Source: three-view drawing plus pictorial views. Frame: mm from the lowest corner of the part. A direction names the side the tool comes from. Give positions to 0.01 mm unless a question says otherwise; leave off trailing zeros. Write each loop counter-clockwise with the first axis right and the second up, starting at its lowest first coordinate (ties: lowest second). Pieces come first, ordered by that corner, then holes. Notation, with made-up numbers: (-33.75, 87) - (-9.75, 87) arc R28 cw to (-9.75, 113) - close; hole circle Ø2 at (74.25, -31.75). An arc over 180 degrees is marked (long way). One line per question, with ' | ' between items. Start each with the question number.
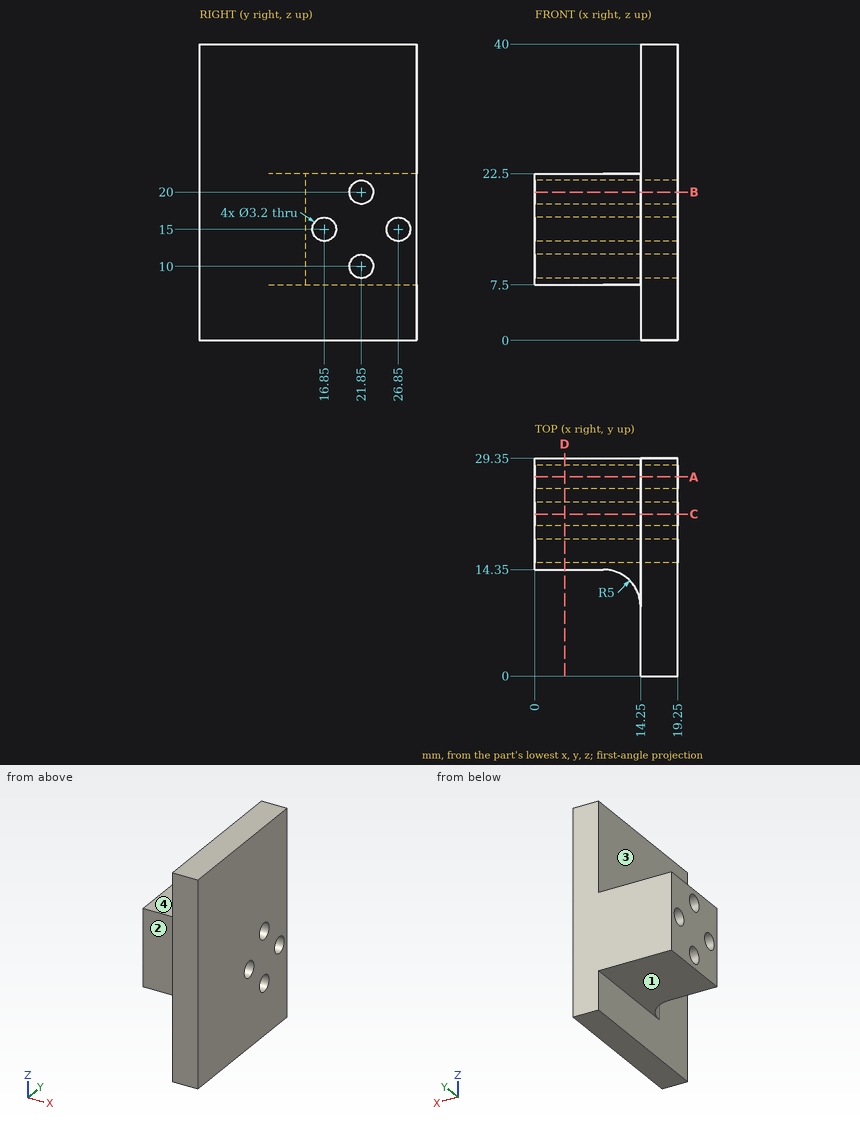
1) Reachability of the marked faces 1, 2, 3 and 4 from +Z, -Z, +X, -X, +Y, -Y: full face, straight path, thin tool, end or side. Return the list, or none.
2) Line query: L1, parallel to Y at x = 7, z = 15; L2, parallel to Y at x = 15.25, z = 15; L3, parallel to Z at x = 11, y = 22.5. Output: solid intervals per line, ascending.
3) Section D-D, the plane x = 4. Output: boundary loops of the cut face in (y, z), plus the area to 3 significant figures.
4) Section A-A, the plane y = 26.85. Output: boundary loops of the cut face in (x, z), plus the area to 3 significant figures.
5) First-contact query: pin 1 Ø3 at (y, z) = (23, 29) entering from -X; pin 2 Ø3 at (y, z) = (16.85, 15) entering from -X; pin 3 Ø7 at (x, y) = (5.5, 22) entering from -Z; pin 4 Ø8 at (x, y) = (3, 22.5) entering from +Z. Flat tips, straight axial feed; report the tip coordinate or a pass-through.
6) Section B-B, the plane z = 20. Output: boundary loops of the cut face in (x, y).
7) Section C-C, the plane y = 21.85. Output: boundary loops of the cut face in (x, z).
Answer key:
1) face 1: -Z, -X, +Y, -Y | face 2: +Z, -Z, -X, -Y | face 3: -X, -Y | face 4: +Z, -X, +Y, -Y
2) L1: 14.35 to 15.25, 18.45 to 25.25, 28.45 to 29.35 | L2: 0 to 15.25, 18.45 to 25.25, 28.45 to 29.35 | L3: 7.5 to 8.54, 11.46 to 18.54, 21.46 to 22.5
3) outline: (14.35, 7.5) - (29.35, 7.5) - (29.35, 22.5) - (14.35, 22.5) - close; hole circle Ø3.2 at (16.85, 15); hole circle Ø3.2 at (21.85, 10); hole circle Ø3.2 at (21.85, 20); hole circle Ø3.2 at (26.85, 15) | area: 193 mm^2
4) outline: (0, 7.5) - (14.25, 7.5) - (14.25, 0) - (19.25, 0) - (19.25, 13.4) - (0, 13.4) - close; (0, 16.6) - (19.25, 16.6) - (19.25, 40) - (14.25, 40) - (14.25, 22.5) - (0, 22.5) - close | area: 352 mm^2
5) pin 1: x = 14.25 | pin 2: through | pin 3: z = 7.5 | pin 4: z = 22.5
6) outline: (0, 14.35) - (9.25, 14.35) arc R5 cw to (14.25, 9.35) - (14.25, 0) - (19.25, 0) - (19.25, 20.25) - (0, 20.25) - close; (0, 23.45) - (19.25, 23.45) - (19.25, 29.35) - (0, 29.35) - close
7) outline: (0, 7.5) - (14.25, 7.5) - (14.25, 0) - (19.25, 0) - (19.25, 8.4) - (0, 8.4) - close; (0, 11.6) - (19.25, 11.6) - (19.25, 18.4) - (0, 18.4) - close; (0, 21.6) - (19.25, 21.6) - (19.25, 40) - (14.25, 40) - (14.25, 22.5) - (0, 22.5) - close
